Autodesk Inventor part; units mm, degrees
ref_plane "YZ Plane" through (0, 0, 0) normal (1, 0, 0) x (0, 1, 0)
ref_plane "XZ Plane" through (0, 0, 0) normal (0, 1, 0) x (-1, 0, 0)
ref_plane "XY Plane" through (0, 0, 0) normal (0, 0, 1) x (1, 0, 0)
sketch "Sketch1" plane through (0, 0, 0) normal (0, 1, 0) x (-1, 0, 0)
  line L0 (14.9, 14.9) -> (-14.9, 14.9)
  line L1 (-14.9, 14.9) -> (-14.9, -14.9)
  line L2 (-14.9, -14.9) -> (14.9, -14.9)
  line L3 (14.9, -14.9) -> (14.9, 14.9)
  point P0 (0, 0)
  dimension "d0" = 29.8
  dimension "d1" = 29.8
  dimension "d2" = 14.9
  dimension "d3" = 14.9
extrude "Extrusion1" add sketch "Sketch1" along normal blind 2
sketch "Sketch2" plane through (0, 2, 0) normal (0, 1, 0) x (1, 0, 0)
  line L0 (-5.715, -5.715) -> (5.715, -5.715)
  line L1 (5.715, -5.715) -> (5.715, 5.715)
  line L2 (5.715, 5.715) -> (-5.715, 5.715)
  line L3 (-5.715, 5.715) -> (-5.715, -5.715)
  line L4 (-4.715, -4.715) -> (4.715, -4.715)
  line L5 (4.715, -4.715) -> (4.715, 4.715)
  line L6 (4.715, 4.715) -> (-4.715, 4.715)
  line L7 (-4.715, 4.715) -> (-4.715, -4.715)
  line L8 (14.9, 14.9) -> (-14.9, 14.9)
  point P0 (0, 0)
  dimension "d6" = 11.43
  dimension "d7" = 11.43
  dimension "d8" = 5.715
  dimension "d9" = 5.715
  dimension "d10" = 1
  dimension "d11" = 1
  dimension "d12" = 1
  dimension "d13" = 1
  dimension "d18" = 9.185
extrude "Extrusion2" add sketch "Sketch2" along normal blind 10
sketch "Sketch3" plane through (0, 2, 0) normal (0, 1, 0) x (1, 0, 0)
  line L0 (4.715, 4.715) -> (-4.715, 4.715)
  line L1 (4.715, -4.715) -> (4.715, 4.715)
  line L2 (-4.715, 4.715) -> (4.715, 4.715)
  line L3 (4.715, 4.715) -> (4.715, -4.715)
  line L4 (4.715, -4.715) -> (-4.715, -4.715)
  line L5 (-4.715, -4.715) -> (-4.715, 4.715)
  point P0 (0, 0)
extrude "Extrusion3" cut sketch "Sketch3" against normal blind 10
equation "\"d1\" = d0"
equation "\"d7\" = d6"
properties part number "Motor_Key_Bearing_3_3"
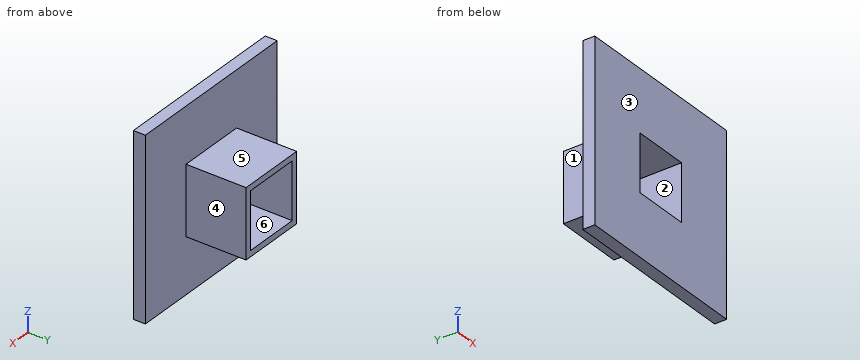
The listing builds one solid part. Answer for the finished solid, in the listing's coordinates (mm). Face numbers are marked on the shaded views. A direction names the side the tool comes from. Coordinates: 2 decimals unless noted, no trailing zeros. Order: outer loops, then holes, each group sorted by start corner. A loop starts at its lowest first (then second) coordinate and runs counter-clockwise, first axis right, second up.
Q1. A cutting plane is placed at B-B, the plane z = 3.5. Write down the section's boundary in (x, y) (3 decimals), and give its area (3 significant figures).
Q2. A cutting plane is placed at C-C, the plane y = 4. Write down the section's boundary in (x, z) (3 decimals).
Q3. Consider line 1 (X direction, y = 8.5, z = -4) (3 decimals); line 2 (Y direction, x = -11.25, z = 12). Determine where each line is inside the solid, lowest interval first.
Q4. For a pull along X with two mould halves and no side action, classify the marked faces 4, 5 and 6 as pulls with the +X half, pulls with the -X half, needs draft (parallel to the pull), parting line crosses it, or undercut.
Q5. Which of the six approach directions +Z, -Z, +X, -X, +Y, -Y give full straight-line access (tool end or side, diameter ignored) to the marked faces 1, 2 and 3?
Q6. Given P1, Ø3, axis at y = 5, z = -2, coming from the -X side (3 decimals); P2, Ø3, axis at x = -2.5, y = 7, coming from the +Z side (3 decimals); P3, Ø4, axis at y = 8, z = -2.5, coming from the +X side (3 decimals), each flat-ended and moving along its own axis, determine where each tip first touches the part or whether it passes through.
Q7. A cutting plane is placed at A-A, the plane x = -4. Write down the section's boundary in (y, z) (3 decimals).
Q8. A cutting plane is placed at D-D, the plane x = -12. Write down the section's boundary in (y, z).
Answers follow:
1. outline: (-14.9, 0) - (-4.715, 0) - (-4.715, 12) - (-5.715, 12) - (-5.715, 2) - (-14.9, 2) - close; (4.715, 0) - (14.9, 0) - (14.9, 2) - (5.715, 2) - (5.715, 12) - (4.715, 12) - close
1. area: 60.7 mm2
2. outline: (-5.715, -5.715) - (5.715, -5.715) - (5.715, 5.715) - (-5.715, 5.715) - close; hole (-4.715, -4.715) - (4.715, -4.715) - (4.715, 4.715) - (-4.715, 4.715) - close
3. line 1: x = -5.715 to -4.715, 4.715 to 5.715
3. line 2: y = 0 to 2
4. face 4: pulls with the +X half
4. face 5: needs draft
4. face 6: undercut
5. face 1: +Z, -Z, -X, +Y
5. face 2: +Y, -Y
5. face 3: +Z, -Z, +X, -X, -Y
6. P1: stops at x = -5.715
6. P2: stops at z = 5.715
6. P3: stops at x = 5.715
7. outline: (0, -14.9) - (2, -14.9) - (2, -5.715) - (12, -5.715) - (12, -4.715) - (0, -4.715) - close; (0, 4.715) - (12, 4.715) - (12, 5.715) - (2, 5.715) - (2, 14.9) - (0, 14.9) - close
8. outline: (0, -14.9) - (2, -14.9) - (2, 14.9) - (0, 14.9) - close
